Verification items for this drawing (mm, ordinates from the low corner). Coordinates: 2 decimals unless noted, no trailing zeros. Order: outer loops, then holes, each group sorted by start corner. A loop starts at its lowest first (then second) coordinate and runs counter-clockwise, first axis right, second up.
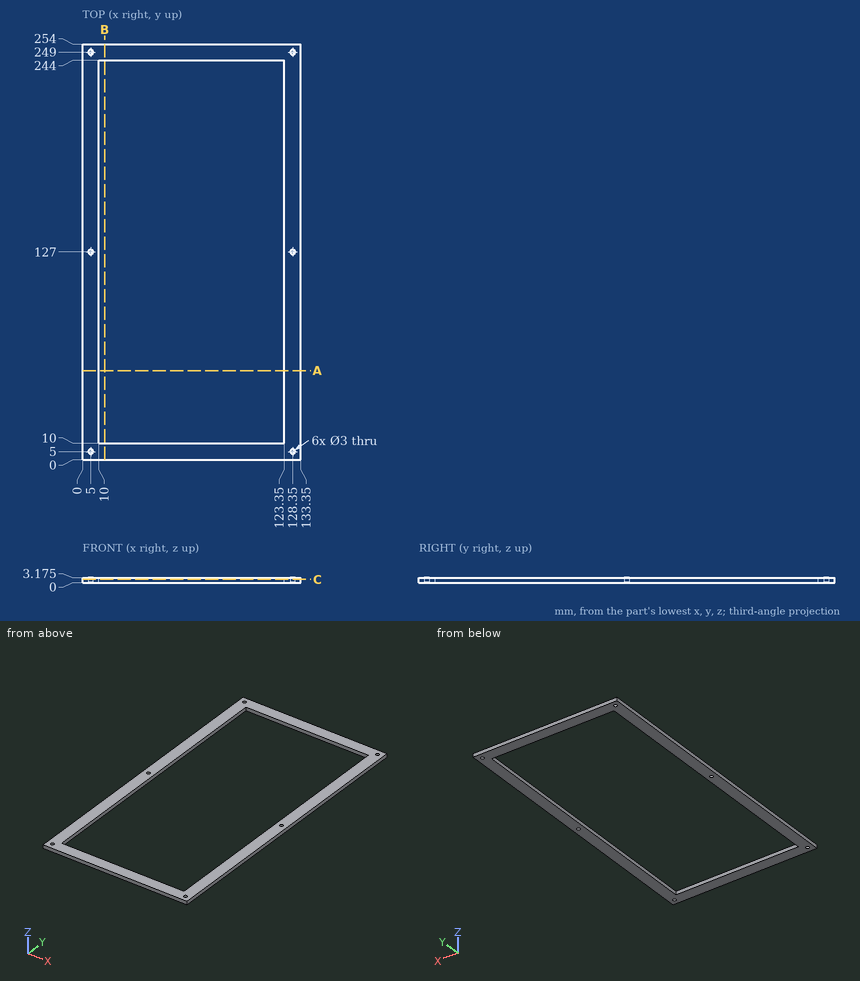
(1) Cross-section at A-A (y = 54.5). Enter the section's corners in (x, z) (3 decimals), and give its area (3 significant figures).
Filled in:
outline: (0, 0) - (10, 0) - (10, 3.175) - (0, 3.175) - close; (123.35, 0) - (133.35, 0) - (133.35, 3.175) - (123.35, 3.175) - close
area: 63.5 mm2
(2) Thickness scan on probe 1 along X at (y, z) = (249, 1.55); probe 2 along Y at (x, z) = (128.35, 1.9); probe 3 along Y at (x, z) = (26.5, 2.15). Record the ranges inside material, lowest first.
Filled in:
probe 1: x = 0 to 3.5, 6.5 to 126.85, 129.85 to 133.35
probe 2: y = 0 to 3.5, 6.5 to 125.5, 128.5 to 247.5, 250.5 to 254
probe 3: y = 0 to 10, 244 to 254
(3) Cross-section at B-B (x = 13.5). Enter the section's corners in (y, z) (3 decimals), and give its area (3 significant figures).
Filled in:
outline: (0, 0) - (10, 0) - (10, 3.175) - (0, 3.175) - close; (244, 0) - (254, 0) - (254, 3.175) - (244, 3.175) - close
area: 63.5 mm2
(4) Cross-section at C-C (z = 2.15). Enter the section's corners in (x, y), and give its area (3 significant figures).
Filled in:
outline: (0, 0) - (133.35, 0) - (133.35, 254) - (0, 254) - close; hole circle Ø3 at (5, 5); hole circle Ø3 at (5, 127); hole circle Ø3 at (5, 249); hole (10, 10) - (123.35, 10) - (123.35, 244) - (10, 244) - close; hole circle Ø3 at (128.35, 5); hole circle Ø3 at (128.35, 127); hole circle Ø3 at (128.35, 249)
area: 7,300 mm2
